Read the model definition and answer for the solid it produces. Units are mm, in the model's axes. Face numbers are marked on the shaded views. A direction names the side the tool comes from. Round coordinates to 2 decimals unless told otherwise and drop trailing zeros. Order: outer loops, then holes, each group sorted by start corner. A loop starts at its lowest first (then second) coordinate and runs counter-clockwise, first axis right, second up. Notation, with made-up numbers: (45.25, -6.5) -> (99.25, -6.5) arc R23 ccw to (99.25, 12.5) -> close; hole circle Ø10 at (36, 67.5). An arc over 180 degrees is marked (long way). Use a Markdown table: item, result. Add a question column.
1. For the marked faces 1, 2, 3, 4 and 5, determine the directions among +Z, -Z, +X, -X, +Y, -Y from which every point of the face is accessible in a straight line to the end or side of a thin tool.
2. Section D-D, the plane z = 8 is taken. Give the vertices of the cut face in (x, y).
3. Section A-A, the plane x = 8 is taken. Give the vertices of the cut face in (y, z), then the cut area to 3 significant figures.
4. Section B-B, the plane y = 0 is taken. Give the vertices of the cut face in (x, z), then the cut area to 3 significant figures.
5. Section C-C, the plane z = 47 is taken. Give the vertices of the cut face in (x, y).
6. The mould has two halves that part along X. Classify the marked faces 6, 7 and 8: +X half, -X half, draft (parallel to the pull), parting line (faces both ways), or undercut.
7. Given pin 1 (2 mm diameter, centred on y = 3.5, z = 26, fed in from +X); pin 2 (4 mm diameter, centred on y = -5.5, z = 44.5, fed in from +X); pin 3 (12 mm diameter, centred on y = -5, z = 39, fed in from +X), each flat-ended and moving along its own axis, determine where each tip first touches the part or whether it passes through.
8. Consider L1, parallel to Y at x = 0, z = 40.5; L2, parallel to Z at x = 3.5, y = -1; L3, parallel to Z at x = 6, y = -2.25. Determine where each line is inside the solid, lowest interval first. Write a range as [from, to].
```python
from build123d import *

# Parameters (mm, degrees)
ESQUISSE1_R             = 10
BOSS_EXTRU_1_DEPTH      = 10
ESQUISSE2_R             = 6
BOSS_EXTRU_2_DEPTH      = 40
ESQUISSE3_R             = 5
ENL_V_MAT_EXTRU_1_DEPTH = 30
ESQUISSE5_W             = 5
ESQUISSE5_H             = 5
ENL_V_MAT_EXTRU_2_DEPTH = 5


with BuildPart() as part:
    # Esquisse1 → Boss.-Extru.1 (new body)
    with BuildSketch(Plane.XY):
        Circle(ESQUISSE1_R)
    extrude(amount=BOSS_EXTRU_1_DEPTH)

    # Esquisse2 → Boss.-Extru.2 (add)
    with BuildSketch(Plane.XY.offset(10)):
        Circle(ESQUISSE2_R)
    extrude(amount=BOSS_EXTRU_2_DEPTH)

    # Esquisse3 → Enlèv. mat.-Extru.1 (cut)
    with BuildSketch(Plane.XY.offset(50)):
        Circle(ESQUISSE3_R)
    extrude(amount=-ENL_V_MAT_EXTRU_1_DEPTH, mode=Mode.SUBTRACT)

    # Esquisse5 → Enlèv. mat.-Extru.2 (cut)
    with BuildSketch(Plane(origin=(0, 0, 0), x_dir=(-1, 0, 0), z_dir=(0, 0, -1))):
        with BuildLine():
            Line((-2.5, 9.682458366), (-2.5, 2.5))
            Line((-2.5, 2.5), (2.5, 2.5))
            Line((2.5, 2.5), (2.5, 9.682458366))
            ThreePointArc((2.5, 9.682458366), (1.260042925, 9.920296963), (0, 10))
            ThreePointArc((0, 10), (-1.260042925, 9.920296963), (-2.5, 9.682458366))
        make_face()
        with BuildLine():
            Line((-2.5, 2.5), (-9.682458366, 2.5))
            ThreePointArc((-9.682458366, 2.5), (-9.920296963, 1.260042925), (-10, 0))
            ThreePointArc((-10, 0), (-9.920296963, -1.260042925), (-9.682458366, -2.5))
            Line((-9.682458366, -2.5), (-2.5, -2.5))
            Line((-2.5, -2.5), (-2.5, 2.5))
        make_face()
        Rectangle(ESQUISSE5_W, ESQUISSE5_H)
        with BuildLine():
            Line((9.682458366, 2.5), (2.5, 2.5))
            Line((2.5, 2.5), (2.5, -2.5))
            Line((2.5, -2.5), (9.682458366, -2.5))
            ThreePointArc((9.682458366, -2.5), (9.920296963, -1.260042925), (10, 0))
            ThreePointArc((10, 0), (9.920296963, 1.260042925), (9.682458366, 2.5))
        make_face()
        with BuildLine():
            Line((2.5, -2.5), (-2.5, -2.5))
            Line((-2.5, -2.5), (-2.5, -9.682458366))
            ThreePointArc((-2.5, -9.682458366), (-1.260042925, -9.920296963), (0, -10))
            ThreePointArc((0, -10), (1.260042925, -9.920296963), (2.5, -9.682458366))
            Line((2.5, -9.682458366), (2.5, -2.5))
        make_face()
    extrude(amount=-ENL_V_MAT_EXTRU_2_DEPTH, mode=Mode.SUBTRACT)


solid = part.part
```
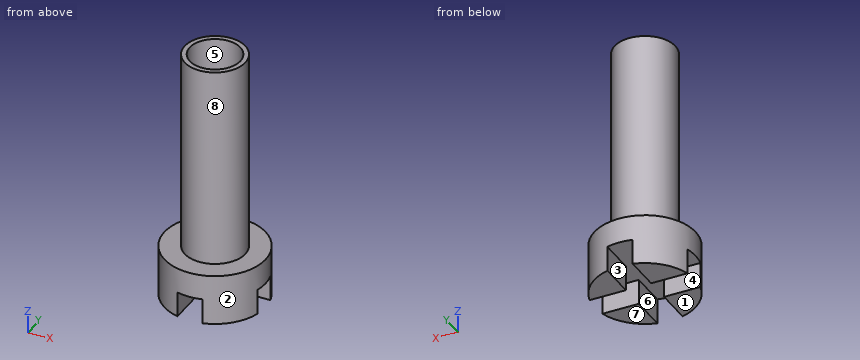
Verdict:
| question | item | result |
|---|---|---|
| 1 | face 1 | -Z, +X, -X, +Y, -Y |
| 1 | face 2 | +Z, -Z |
| 1 | face 3 | -Z, +Y, -Y |
| 1 | face 4 | -Z, +X, -X |
| 1 | face 5 | +Z |
| 2 | outline | circle Ø20 at (0, 0) |
| 3 | outline | (-6, 0) -> (-2.5, 0) -> (-2.5, 5) -> (2.5, 5) -> (2.5, 0) -> (6, 0) -> (6, 10) -> (-6, 10) -> close |
| 3 | area | 95.0 mm2 |
| 4 | outline | (-10, 5) -> (10, 5) -> (10, 10) -> (6, 10) -> (6, 50) -> (5, 50) -> (5, 20) -> (-5, 20) -> (-5, 50) -> (-6, 50) -> (-6, 10) -> (-10, 10) -> close |
| 4 | area | 280 mm2 |
| 5 | outline | circle Ø12 at (0, 0); hole circle Ø10 at (0, 0) |
| 6 | face 6 | undercut |
| 6 | face 7 | draft |
| 6 | face 8 | parting line |
| 7 | pin 1 | stops at x = 5.45 |
| 7 | pin 2 | stops at x = 4.87 |
| 7 | pin 3 | stops at x = 6 |
| 8 | L1 | y = [-6, -5], [5, 6] |
| 8 | L2 | z = [5, 20] |
| 8 | L3 | z = [5, 10] |
